Check sheet for the modelled part. Datum: model origin and axes. Units: mm. A direction names the side the tool comes from. Round coordinates to 2 decimals unless told otherwise and drop trailing zeros. Write each loop counter-clockwise with the first axis right and the second up, starting at its lowest first coordinate (ties: lowest second). Pieces come first, ordered by that corner, then holes. Notation, with made-up numbers: (50.5, 74.25) - (63.5, 74.25) arc R27 ccw to (63.5, 95.25) - close; hole circle Ø6 at (-4, 43). An arc over 180 degrees is marked (long way). Answer as a JSON object with one key per item and string values. Group by question number.
Item 1: Sectioned sample at D-D on y = 18. Record the boundary of the cut face in (x, z), plus the area to 3 significant figures.
Item 2: Set-up check for faces 5 (the flat face through (-29, 16.55, 11)), 6 (the flat face through (-71.82, -19.18, 15.71)), 7 (the flat face through (-76, 4.138, 11)), 8 (the flat face through (-25, -32.764, 11)): record each of +Z, -Z, +X, -X, +Y, -Y from which the full face is reachable in a straight line by a thin tool's end or side.
Item 3: Sectioned sample at B-B on y = -22. Record the boundary of the cut face in (x, z).
Item 4: Release check for a two-part mould opening along X. For faces 1 (the cylindrical face through (-59.528, 6.836, 10.846)), 2 (the flat face through (-62.147, -37, 11)), 3 (the flat face through (-66.351, 16, 21)), 4 (the flat face through (-74, -41.85, 11)) record: pulls with the +X half, pulls with the -X half, needs draft (parallel to the pull), parting line crosses it, or undercut.
Item 5: Thickness scan on line 1 (X direction, y = -13.5, z = 16); line 2 (Y direction, x = -30.5, z = 11.75); line 3 (X direction, y = -36.5, z = 20.5). Record the ranges inside material, lowest first.
Item 6: Gauge pin test, flat ends, axial feed: P1, Ø5, axis at x = -20.5, z = 19.5, coming from the -Y side; P2, Ø2.5, axis at y = -38, z = 11, coming from the +X side; P3, Ø1.9, axis at y = 10.5, z = 20.5, coming from the -X side; P4, Ø9.5, axis at x = -71, z = 15.5, coming from the +Y side. Record the tip position at first contact, or that the pin passes through.
Item 7: Sectioned sample at A-A on z = 16. Record the boundary of the cut face in (x, y), plus the area to 3 significant figures.
Item 8: Sectioned sample at C-C on x = -16. Record the boundary of the cut face in (y, z), plus the area to 3 significant figures.
```python
from build123d import *

# Parameters (mm, degrees)
F0_R     = 12.235382
F0_R_2   = 6.56791
F1_DEPTH = 22
F3_DEPTH = 68.400986
F4_R     = 6.772797
F5_DEPTH = 10


with BuildPart() as f1:
    # F0 (on Top) → F1 (new body)
    with BuildSketch(Plane.XY):
        Polygon((-62.147137, -32.764492), (13.882609, -32.764492), (13.882609, 26.550179), (-66.351078, 26.550179), (-66.351078, 4.138138), (-66.351078, -32.764492), align=None)
        with Locations((-16.783873, -13.015332)):
            Circle(F0_R, mode=Mode.SUBTRACT)
        with Locations((-52.966461, 6.546799)):
            Circle(F0_R_2, mode=Mode.SUBTRACT)
        Polygon((-62.147137, -41.849807), (-62.147137, -32.764492), (-66.351078, -32.764492), (-66.351078, 4.138138), (-85.250083, 4.138138), (-85.250083, -41.849807), align=None)
    extrude(amount=F1_DEPTH)

    # F2 (on face) → F3 (cut, through all)
    with BuildSketch(Plane.XZ.offset(41.849807)):
        Polygon((-69.480886, 11.999899), (-65.448255, 19.663964), (-74.101845, 19.324293), align=None)
    extrude(amount=-F3_DEPTH, mode=Mode.SUBTRACT)

    # F4 (on face) → F5 (cut)
    with BuildSketch(Plane(origin=(0, 26.550179, 0), x_dir=(-1, 0, 0), z_dir=(0, 1, 0))):
        with Locations((29.194595, 10.745674)):
            Circle(F4_R)
    extrude(amount=-F5_DEPTH, mode=Mode.SUBTRACT)


solid = f1.part
```
Completed:
{
 "1": {"outline": "(-66.35, 0) - (13.88, 0) - (13.88, 22) - (-66.35, 22) - (-66.35, 19.63) - (-65.45, 19.66) - (-66.35, 17.95) - close; hole circle Ø13.55 at (-29.19, 10.75)", "area": "1,620 mm²"},
 "2": {"face 5": "+Y", "face 6": "+Y, -Y", "face 7": "+Z, -Z, -X, +Y", "face 8": "+Z, -Z, +X, -Y"},
 "3": {"outline": "(-85.25, 0) - (-25.09, 0) - (-25.09, 22) - (-85.25, 22) - close; (-8.48, 0) - (13.88, 0) - (13.88, 22) - (-8.48, 22) - close; hole (-74.1, 19.32) - (-69.48, 12) - (-65.45, 19.66) - close"},
 "4": {"face 1": "undercut", "face 2": "pulls with the +X half", "face 3": "pulls with the -X half", "face 4": "needs draft"},
 "5": {"line 1": "-85.25 to -72, -67.38 to -29.01, -4.56 to 13.88", "line 2": "-32.76 to 16.55", "line 3": "-85.25 to -62.15"},
 "6": {"P1": "y = -32.76", "P2": "x = -62.15", "P3": "x = -66.35", "P4": "y = 26.55"},
 "7": {"outline": "(-85.25, -41.85) - (-72, -41.85) - (-72, 4.14) - (-85.25, 4.14) - close; (-67.38, -41.85) - (-62.15, -41.85) - (-62.15, -32.76) - (13.88, -32.76) - (13.88, 26.55) - (-24.92, 26.55) - (-24.92, 16.55) - (-33.47, 16.55) - (-33.47, 26.55) - (-66.35, 26.55) - (-66.35, 4.14) - (-67.38, 4.14) - close; hole circle Ø13.14 at (-52.97, 6.55); hole circle Ø24.47 at (-16.78, -13.02)", "area": "4,760 mm²"},
 "8": {"outline": "(-32.76, 0) - (-25.23, 0) - (-25.23, 22) - (-32.76, 22) - close; (-0.81, 0) - (26.55, 0) - (26.55, 22) - (-0.81, 22) - close", "area": "768 mm²"}
}
